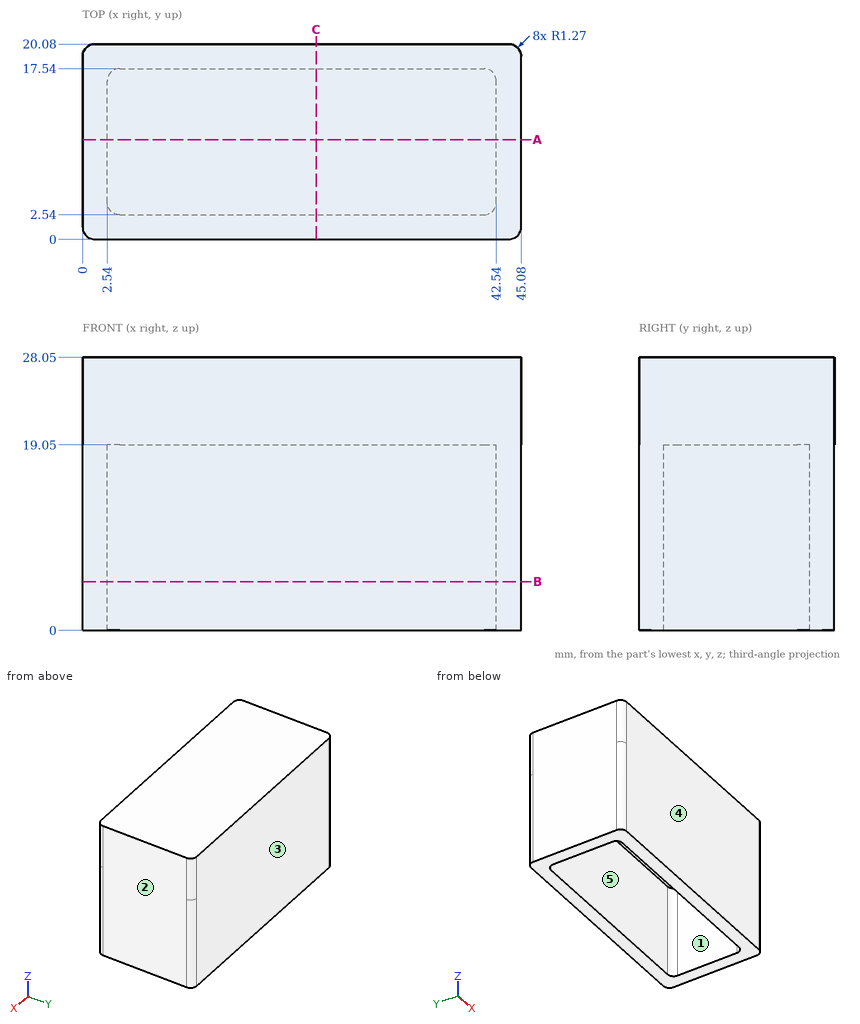
Could you check a few things on this drawing? It's one solid part, dimensions in mm from its lowest x, y, z. A direction names the side the tool comes from. Coordinates: 2 decimals unless noted, no trailing zeros. Loops run counter-clockwise (first coordinate to the right, second up) from the corner with the lowest first, then second, coordinate; pieces in that order, holes last. Notation, with made-up numbers: (43.5, -37) - (51.5, -37) arc R20 ccw to (51.5, -27) - close; hole circle Ø6 at (67, 79). An arc over 180 degrees is marked (long way). Return JSON: item names as keys, results as strings. Group by question number.
Item 1: If we section it at C-C on x = 24: Write out the boundary of the cut face in (y, z).
Item 2: If we section it at B-B on z = 5: Write out the boundary of the cut face in (x, y), and give its area (3 significant figures).
Item 3: We'd pull the mould along X, two halves only. Please class the marked faces 1, 2 and 3: +X half, -X half, draft (parallel to the pull), parting line (faces both ways), or undercut.
Item 4: On a 3-axis mill with a long thin cutter (end or side, diameter ignored), from which of +Z, -Z, +X, -X, +Y, -Y can I reach the whole of each face in a straight line? I mean the marked faces 4 and 5. Say none if no direction works.
Item 5: If we section it at A-A on y = 10.25: Write out the boundary of the cut face in (x, z).
Item 6: Will these pins go through, and if not, where does the flat tip stop? P1, Ø6, axis at x = 32, y = 13, coming from the -Z side; P2, Ø6, axis at x = 36, y = 5.5, coming from the -Z side.
Item 7: I need wall thicknesses on line 1 (Y direction, x = 35.5, z = 11.5); line 2 (X direction, y = 6.5, z = 3); line 3 (X direction, y = 17, z = 4.25). Which ranges of each line are inside material? Lowest first, please. Write a range as from..to.
Calculated:
{
 "1": {"outline": "(0, 0) - (2.54, 0) - (2.54, 19.05) - (17.54, 19.05) - (17.54, 0) - (20.08, 0) - (20.08, 28.05) - (0, 28.05) - close"},
 "2": {"outline": "(0, 1.27) arc R1.27 ccw to (1.27, 0) - (43.81, 0) arc R1.27 ccw to (45.08, 1.27) - (45.08, 18.81) arc R1.27 ccw to (43.81, 20.08) - (1.27, 20.08) arc R1.27 ccw to (0, 18.81) - close; hole (2.54, 3.81) arc R1.27 ccw to (3.81, 2.54) - (41.27, 2.54) arc R1.27 ccw to (42.54, 3.81) - (42.54, 16.27) arc R1.27 ccw to (41.27, 17.54) - (3.81, 17.54) arc R1.27 ccw to (2.54, 16.27) - close", "area": "305 mm^2"},
 "3": {"face 1": "undercut", "face 2": "+X half", "face 3": "draft"},
 "4": {"face 4": "+Z, -Z, +X, -X, -Y", "face 5": "-Z"},
 "5": {"outline": "(0, 0) - (2.54, 0) - (2.54, 19.05) - (42.54, 19.05) - (42.54, 0) - (45.08, 0) - (45.08, 28.05) - (0, 28.05) - close"},
 "6": {"P1": "stops at z = 19.05", "P2": "stops at z = 0"},
 "7": {"line 1": "y = 0..2.54, 17.54..20.08", "line 2": "x = 0..2.54, 42.54..45.08", "line 3": "x = 0..2.77, 42.31..45.08"}
}
